```python
from build123d import *

# Parameters (mm, degrees)
SKETCH1_W           = 33
SKETCH1_H           = 47
SKETCH1_R           = 1.75
SKETCH1_W_2         = 27
SKETCH1_H_2         = 27
BOSS_EXTRUDE1_DEPTH = 8
SKETCH3_W           = 27
SKETCH3_H           = 27
BOSS_EXTRUDE2_DEPTH = 6
CHAMFER1_SIZE       = 2
SKETCH4_R           = 1.5
CUT_EXTRUDE1_DEPTH  = 10
SKETCH5_W           = 4
SKETCH5_H           = 25
CUT_EXTRUDE2_DEPTH  = 3
CUT_EXTRUDE3_DEPTH  = 3


with BuildPart() as part:
    # Sketch1 → Boss-Extrude1 (new body)
    with BuildSketch(Plane.XY):
        with Locations((16.5, 23.5)):
            Rectangle(SKETCH1_W, SKETCH1_H)
        with Locations((16.5, 42)):
            Circle(SKETCH1_R, mode=Mode.SUBTRACT)
        with Locations((16.5, 5)):
            Circle(SKETCH1_R, mode=Mode.SUBTRACT)
        with Locations((16.5, 23.5)):
            Rectangle(SKETCH1_W_2, SKETCH1_H_2, mode=Mode.SUBTRACT)
    extrude(amount=BOSS_EXTRUDE1_DEPTH)

    # Sketch3 → Boss-Extrude2 (add)
    with BuildSketch(Plane(origin=(0, 0, 0), x_dir=(-1, 0, 0), z_dir=(0, 0, -1))):
        with Locations((-16.5, 23.5)):
            Rectangle(SKETCH3_W, SKETCH3_H)
    extrude(amount=-BOSS_EXTRUDE2_DEPTH)

    # Chamfer1
    chamfer1_edges = [part.edges().sort_by_distance(p)[0] for p in [
        (14.75, 42, 8),
        (14.75, 5, 8),
    ]]
    chamfer(chamfer1_edges, length=CHAMFER1_SIZE)

    # Sketch4 → Cut-Extrude1 (cut)
    with BuildSketch(Plane.XY.offset(6)):
        with Locations((6.5, 33.5)):
            Circle(SKETCH4_R)
        with Locations((6.25, 13.501562561)):
            Circle(SKETCH4_R)
    extrude(amount=-CUT_EXTRUDE1_DEPTH, mode=Mode.SUBTRACT)

    # Sketch5 → Cut-Extrude2 (cut)
    with BuildSketch(Plane.XY.offset(6)):
        with Locations((27, 23.5)):
            Rectangle(SKETCH5_W, SKETCH5_H)
    extrude(amount=-CUT_EXTRUDE2_DEPTH, mode=Mode.SUBTRACT)

    # Sketch6 → Cut-Extrude3 (cut)
    with BuildSketch(Plane(origin=(0, 0, 0), x_dir=(-1, 0, 0), z_dir=(0, 0, -1))):
        Polygon((-6.5, 36.964101615), (-9.5, 35.232050808), (-9.5, 31.767949192), (-6.5, 30.035898385), (-3.5, 31.767949192), (-3.5, 35.232050808), align=None)
        Polygon((-3.25, 15.233613369), (-6.25, 16.965664176), (-9.25, 15.233613369), (-9.25, 11.769511753), (-6.25, 10.037460946), (-3.25, 11.769511753), align=None)
    extrude(amount=-CUT_EXTRUDE3_DEPTH, mode=Mode.SUBTRACT)


solid = part.part
```
Check sheet for the modelled part. Datum: model origin and axes. Units: mm. A direction names the side the tool comes from. Give positions to 0.01 mm unless a question says otherwise; leave off trailing zeros. Order: outer loops, then holes, each group sorted by start corner. A loop starts at its lowest first (then second) coordinate and runs counter-clockwise, first axis right, second up. Notation, with made-up numbers: (51, 7.25) -> (83, 7.25) arc R21 ccw to (83, 34.25) -> close; hole circle Ø6 at (58.25, 24). An arc over 180 degrees is marked (long way). Use CSV: the item, a comma, the result in double quotes. Start each with the question number.
1) Sectioned sample at A-A, the plane y = 33.5. Record the boundary of the cut face in (x, z), plus the area to 3 significant figures.
2) Sectioned sample at B-B, the plane z = 2. Record the boundary of the cut face in (x, y).
3) Sectioned sample at C-C, the plane x = 27. Record the boundary of the cut face in (y, z).
4) Material ranges on line 1 (Y direction, x = 16.5, z = 2.7); line 2 (X direction, y = 15.5, z = 3.5); line 3 (Y direction, x = 6.25, z = 3.95), recorded low to high. Write a range as from..to.
5) Go/stop test with flat-tipped pins: P1, Ø13.5, axis at x = 16, y = 17.5, coming from the +Z side; P2, Ø4, axis at x = 6.25, y = 13.5, coming from the -Z side. Record where each tip stops, or that it passes through.
6) Sectioned sample at D-D, the plane z = 4.25. Record the boundary of the cut face in (x, y).
7) Set-up check for faces 4 (the face through (27, 24, 3)), 5 (the face through (6.175, 32.036, 4.521)), 6 (the face through (4.73, 16.09, 1.48)): record each of +Z, -Z, +X, -X, +Y, -Y from which the full face is reachable in a straight line by a thin tool's end or side.
8) Mould release check, pull along X, two halves, no side actions. Record for faces 1 (the face through (0, 23, 4)), 2 (the face through (17.31, 3.45, 2.96)), 3 (the face through (2, 24, 8)): released by +X, released by -X, zero draft, split by the parting line, or undercut.
Recorded:
1,outline,"(0, 0) -> (3.5, 0) -> (3.5, 3) -> (5, 3) -> (5, 6) -> (3, 6) -> (3, 8) -> (0, 8) -> close; (8, 3) -> (9.5, 3) -> (9.5, 0) -> (33, 0) -> (33, 8) -> (30, 8) -> (30, 6) -> (29, 6) -> (29, 3) -> (25, 3) -> (25, 6) -> (8, 6) -> close"
1,area,"171 mm2"
2,outline,"(0, 0) -> (33, 0) -> (33, 47) -> (0, 47) -> close; hole (3.25, 11.77) -> (6.25, 10.04) -> (9.25, 11.77) -> (9.25, 15.23) -> (6.25, 16.97) -> (3.25, 15.23) -> close; hole (3.5, 31.77) -> (6.5, 30.04) -> (9.5, 31.77) -> (9.5, 35.23) -> (6.5, 36.96) -> (3.5, 35.23) -> close; hole circle Ø3.5 at (16.5, 5); hole circle Ø3.5 at (16.5, 42)"
3,outline,"(0, 0) -> (47, 0) -> (47, 8) -> (37, 8) -> (37, 6) -> (36, 6) -> (36, 3) -> (11, 3) -> (11, 6) -> (10, 6) -> (10, 8) -> (0, 8) -> close"
4,line 1,"0..3.25, 6.75..40.25, 43.75..47"
4,line 2,"0..25, 29..33"
4,line 3,"0..12, 15..32.02, 34.98..47"
5,P1,"z = 6"
5,P2,"z = 3"
6,outline,"(0, 0) -> (33, 0) -> (33, 47) -> (0, 47) -> close; hole circle Ø3 at (6.25, 13.5); hole circle Ø3 at (6.5, 33.5); hole circle Ø3.5 at (16.5, 5); hole circle Ø3.5 at (16.5, 42); hole (25, 11) -> (29, 11) -> (29, 36) -> (25, 36) -> close"
7,face 4,"+Z"
7,face 5,"+Z, -Z"
7,face 6,"-Z"
8,face 1,"released by -X"
8,face 2,"undercut"
8,face 3,"zero draft"
